Verification items for the finished model (mm, model axes). A direction names the side the tool comes from. Round coordinates to 2 decimals unless told otherwise and drop trailing zeros. Loops run counter-clockwise (first coordinate to the right, second up) from the corner with the lowest first, then second, coordinate; pieces in that order, holes last. Notation, with made-up numbers: (71, -37) -> (128, -37) arc R30 ccw to (128, -12) -> close; hole circle Ø9 at (34.25, 52.5). An arc over 180 degrees is marked (long way). Use a Markdown table: item, result. Add a question column.
```python
from build123d import *

# Parameters (mm, degrees)
SKETCH1_R           = 35
SKETCH1_W           = 100
SKETCH1_H           = 30
BOSS_EXTRUDE2_DEPTH = 10
SKETCH2_R           = 3
SKETCH2_R_2         = 1.5
CUT_EXTRUDE2_DEPTH  = 4
SKETCH3_R           = 1.5
CUT_EXTRUDE3_DEPTH  = 112.510800428
SKETCH5_W           = 80
SKETCH5_H           = 8
BOSS_EXTRUDE3_DEPTH = 12
SKETCH6_R           = 1.5
CUT_EXTRUDE4_DEPTH  = 136.260863051
SKETCH7_R           = 1.5
CUT_EXTRUDE5_DEPTH  = 136.260863051


with BuildPart() as part:
    # Sketch1 → Boss-Extrude2 (new body)
    with BuildSketch(Plane.XY):
        Circle(SKETCH1_R)
        with Locations((50, -33.064391539)):
            Rectangle(SKETCH1_W, SKETCH1_H)
        with Locations((-50, 33.318305145)):
            Rectangle(SKETCH1_W, SKETCH1_H)
    extrude(amount=BOSS_EXTRUDE2_DEPTH)

    # Sketch2 → Cut-Extrude2 (cut)
    # profile 1 of 6: a face of its own
    with BuildSketch(Plane.XY.offset(10)):
        with Locations((0, -13.598895475)):
            Circle(SKETCH2_R)
        with Locations((0, -13.598895475)):
            Circle(SKETCH2_R_2, mode=Mode.SUBTRACT)
    # profile 2 of 6: a face of its own
    with BuildSketch(Plane.XY.offset(10)):
        with Locations((-11.776988944, -6.799447737)):
            Circle(SKETCH2_R)
        with Locations((-11.776988944, -6.799447737)):
            Circle(SKETCH2_R_2, mode=Mode.SUBTRACT)
    # profile 3 of 6: a face of its own
    with BuildSketch(Plane.XY.offset(10)):
        with Locations((-11.776988944, 6.799447737)):
            Circle(SKETCH2_R)
        with Locations((-11.776988944, 6.799447737)):
            Circle(SKETCH2_R_2, mode=Mode.SUBTRACT)
    # profile 4 of 6: a face of its own
    with BuildSketch(Plane.XY.offset(10)):
        with Locations((0, 13.598895475)):
            Circle(SKETCH2_R)
        with Locations((0, 13.598895475)):
            Circle(SKETCH2_R_2, mode=Mode.SUBTRACT)
    # profile 5 of 6: a face of its own
    with BuildSketch(Plane.XY.offset(10)):
        with Locations((11.776988944, 6.799447737)):
            Circle(SKETCH2_R)
        with Locations((11.776988944, 6.799447737)):
            Circle(SKETCH2_R_2, mode=Mode.SUBTRACT)
    # profile 6 of 6: a face of its own
    with BuildSketch(Plane.XY.offset(10)):
        with Locations((11.776988944, -6.799447737)):
            Circle(SKETCH2_R)
        with Locations((11.776988944, -6.799447737)):
            Circle(SKETCH2_R_2, mode=Mode.SUBTRACT)
    extrude(amount=-CUT_EXTRUDE2_DEPTH, mode=Mode.SUBTRACT)

    # Sketch3 → Cut-Extrude3 (cut, through all)
    with BuildSketch(Plane.XY.offset(10)):
        with Locations((0, -13.598895475)):
            Circle(SKETCH3_R)
        with Locations((-11.776988944, -6.799447737)):
            Circle(SKETCH3_R)
        with Locations((-11.776988944, 6.799447737)):
            Circle(SKETCH3_R)
        with Locations((0, 13.598895475)):
            Circle(SKETCH3_R)
        with Locations((11.776988944, 6.799447737)):
            Circle(SKETCH3_R)
        with Locations((11.776988944, -6.799447737)):
            Circle(SKETCH3_R)
    extrude(amount=-CUT_EXTRUDE3_DEPTH, mode=Mode.SUBTRACT)

    # Sketch5 → Boss-Extrude3 (add)
    with BuildSketch(Plane.XY.offset(10)):
        with Locations((-60, 44.318305145)):
            Rectangle(SKETCH5_W, SKETCH5_H)
        with Locations((60, -44.064391539)):
            Rectangle(SKETCH5_W, SKETCH5_H)
    extrude(amount=BOSS_EXTRUDE3_DEPTH)

    # Sketch6 → Cut-Extrude4 (cut, through all)
    with BuildSketch(Plane(origin=(0, 40.318305145, 0), x_dir=(-1, 0, 0), z_dir=(0, -1, 0))):
        with Locations(Location((89.985573023, -16, 0), (0, 0, 90))):
            Circle(SKETCH6_R)
        with Locations(Location((59.985573023, -16, 0), (0, 0, 90))):
            Circle(SKETCH6_R)
        with Locations(Location((29.985573023, -16, 0), (0, 0, 90))):
            Circle(SKETCH6_R)
    extrude(amount=-CUT_EXTRUDE4_DEPTH, mode=Mode.SUBTRACT)

    # Sketch7 → Cut-Extrude5 (cut, through all)
    with BuildSketch(Plane(origin=(0, -40.064391539, 0), x_dir=(1, 0, 0), z_dir=(0, 1, 0))):
        with Locations(Location((29.372536894, -16, 0), (0, 0, 180))):
            Circle(SKETCH7_R)
        with Locations(Location((59.372536894, -16, 0), (0, 0, 180))):
            Circle(SKETCH7_R)
        with Locations(Location((89.372536894, -16, 0), (0, 0, 180))):
            Circle(SKETCH7_R)
    extrude(amount=-CUT_EXTRUDE5_DEPTH, mode=Mode.SUBTRACT)


solid = part.part
```
1) Sectioned sample at B-B on z = 3.5. Enter the section's corners in (x, y).
2) Sectioned sample at C-C on y = 24. Enter the section's corners in (x, z).
3) Thickness scan on line 1 (X direction, y = 42.5, z = 16); line 2 (X direction, y = 7.5, z = 7.5); line 3 (Y direction, x = -13, z = 8.5). Record the ranges inside material, lowest first.
4) Sectioned sample at D-D on x = 22. Enter the section's corners in (y, z).
5) Access from +Z, -Z, +X, -X, +Y, -Y to the whole of each face (thin tool, end or side, straight path). Record for faces 1 (the face through (0, -42, 5)), 2 (the face through (0, 42, 5)), 3 (the face through (100, -37, 6)), 4 (the face through (-13, 8, 6)), 5 (the face through (59, -40.064, 19)).
6) Release check for a two-part mould opening along X. For faces 6 (the face through (14.548, -7.948, 8.028)), 7 (the face through (-61, 40.318, 13)), 8 (the face through (-20, 44, 16)), 9 (the face through (14.64, 7.7, 8.03)) record: released by +X, released by -X, zero draft, split by the parting line, or undercut.
7) Sectioned sample at A-A on x = -79. Enter the section's corners in (y, z), then the cut area to 3 significant figures.
8) Go/stop test with flat-tipped pins: pin 1 (10 mm diameter, centred on x = 64, z = 18, fed in from +Y); pin 2 (6.5 mm diameter, centred on x = 1.5, y = -13.5, fed in from +Z); pin 3 (8 mm diameter, centred on x = -54, z = 7, fed in from -Y). Record where each tip stops, or that it passes through.
Geometry results:
| question | item | result |
|---|---|---|
| 1 | outline | (-100, 18.32) -> (-29.82, 18.32) arc R35 ccw to (0, -35) -> (0, -48.06) -> (100, -48.06) -> (100, -18.06) -> (29.98, -18.06) arc R35 ccw to (0, 35) -> (0, 48.32) -> (-100, 48.32) -> close; hole circle Ø3 at (-11.78, -6.8); hole circle Ø3 at (-11.78, 6.8); hole circle Ø3 at (0, -13.6); hole circle Ø3 at (0, 13.6); hole circle Ø3 at (11.78, -6.8); hole circle Ø3 at (11.78, 6.8) |
| 2 | outline | (-100, 0) -> (25.48, 0) -> (25.48, 10) -> (-100, 10) -> close |
| 3 | line 1 | -100 to -91.49, -88.49 to -61.49, -58.49 to -31.49, -28.49 to -20 |
| 3 | line 2 | -34.19 to -14.69, -8.86 to 8.86, 14.69 to 34.19 |
| 3 | line 3 | -32.5 to -9.54, -4.06 to 4.06, 9.54 to 48.32 |
| 4 | outline | (-48.06, 0) -> (27.22, 0) -> (27.22, 10) -> (-40.06, 10) -> (-40.06, 22) -> (-48.06, 22) -> close |
| 5 | face 1 | +Z, -Z, -X, -Y |
| 5 | face 2 | +Z, -Z, +X, +Y |
| 5 | face 3 | +Z, -Z, +X, +Y, -Y |
| 5 | face 4 | +Z |
| 5 | face 5 | +Z, +X, -X, +Y |
| 6 | face 6 | undercut |
| 6 | face 7 | zero draft |
| 6 | face 8 | released by +X |
| 6 | face 9 | undercut |
| 7 | outline | (18.32, 0) -> (48.32, 0) -> (48.32, 22) -> (40.32, 22) -> (40.32, 10) -> (18.32, 10) -> close |
| 7 | area | 396 mm^2 |
| 8 | pin 1 | y = -40.06 |
| 8 | pin 2 | z = 10 |
| 8 | pin 3 | y = 18.32 |
